Design review of the part built by this model. Coordinates are the model's own, in mm. Face numbers are marked on the shaded views. A direction names the side the tool comes from. Coordinates: 2 decimals unless noted, no trailing zeros. Write each loop counter-clockwise with the first axis right and the second up, starting at its lowest first coordinate (ties: lowest second). Pieces come first, ordered by that corner, then holes. Notation, with made-up numbers: (18.5, 67.5) - (49.5, 67.5) arc R6 ccw to (49.5, 76.5) - close; hole circle Ø4 at (-13, 50). An arc over 180 degrees is marked (long way). One line per item, written item: value.
from build123d import *

# Parameters (mm, degrees)
SKETCH5_R           = 4
SKETCH5_R_2         = 11
BOSS_EXTRUDE4_DEPTH = 10
SKETCH5_3_R         = 4
BOSS_EXTRUDE5_DEPTH = 25


with BuildPart() as part:
    # Sketch5 → Boss-Extrude4 (new body)
    with BuildSketch(Plane.XY):
        with BuildLine():
            Line((-20, 125), (-20, -125))
            ThreePointArc((-20, -125), (0, -145), (20, -125))
            Line((20, -125), (20, 125))
            ThreePointArc((20, 125), (0, 145), (-20, 125))
        make_face()
        with Locations((0, -125)):
            Circle(SKETCH5_R, mode=Mode.SUBTRACT)
        with Locations((0, 125)):
            Circle(SKETCH5_R_2, mode=Mode.SUBTRACT)
        with BuildLine():
            Line((-11, 90), (-11, -90))
            ThreePointArc((-11, -90), (0, -101), (11, -90))
            Line((11, -90), (11, 90))
            ThreePointArc((11, 90), (0, 101), (-11, 90))
        make_face(mode=Mode.SUBTRACT)
    extrude(amount=BOSS_EXTRUDE4_DEPTH)

    # Sketch5_3 → Boss-Extrude5 (add)
    with BuildSketch(Plane.XY):
        with Locations((0, -125)):
            Circle(SKETCH5_3_R)
    extrude(amount=BOSS_EXTRUDE5_DEPTH)


solid = part.part
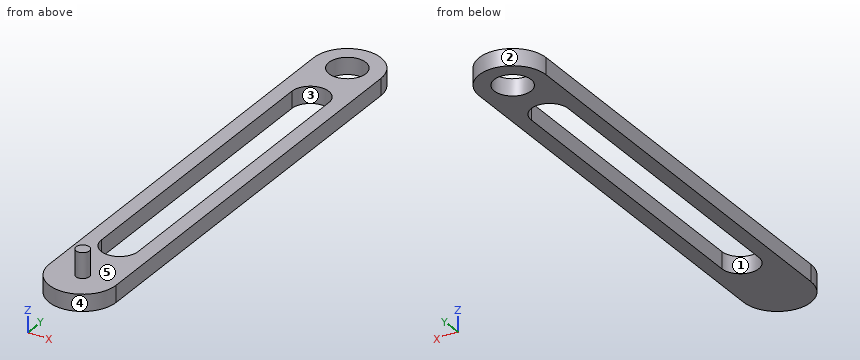
1. Consider section A-A, the plane y = -26. Write out the cut boundary in (x, z), then the cut area to 3 significant figures.
Answer block:
outline: (-20, 0) - (-11, 0) - (-11, 10) - (-20, 10) - close; (11, 0) - (20, 0) - (20, 10) - (11, 10) - close
area: 180 mm^2
2. Mouldability with a two-part tool opening along Y and no side actions: class the marked faces 3, 4 and 5 as released by +Y, released by -Y, zero draft, split by the parting line, or undercut.
Answer block:
face 3: undercut
face 4: released by -Y
face 5: zero draft
3. Consider section D-D, the plane y = 98.5. Write out the cut boundary in (x, z), then the cut area to 3 significant figures.
Answer block:
outline: (-20, 0) - (-6.98, 0) - (-6.98, 10) - (-20, 10) - close; (6.98, 0) - (20, 0) - (20, 10) - (6.98, 10) - close
area: 260 mm^2
4. Consider section C-C, the plane z = 22. Write out the cut boundary in (x, y), then the cut area to 3 significant figures.
Answer block:
outline: circle Ø8 at (0, -125)
area: 50.3 mm^2
5. Wall thickness on line 1 along Y through (x, z) = (0, 2.25); line 2 along X through (y, z) = (30.5, 3.5); line 3 along Y through (x, z) = (-5, 1.25): over which ranges is each line inside the solid? List them lowest first.
Answer block:
line 1: y = -145 to -101, 101 to 114, 136 to 145
line 2: x = -20 to -11, 11 to 20
line 3: y = -144.36 to -99.8, 99.8 to 115.2, 134.8 to 144.36
6. For the marked faces 1 and 2, list the 3-axis set-ups (+Z, -Z, +X, -X, +Y, -Y) from which the entire face can be reached by the end or side of a thin tool; tool diameter is ignored.
Answer block:
face 1: +Z, -Z
face 2: +Z, -Z, +Y
7. Consider section B-B, the plane x = 0. Write out the cut boundary in (y, z), then the cut area to 3 significant figures.
Answer block:
outline: (-145, 0) - (-101, 0) - (-101, 10) - (-121, 10) - (-121, 25) - (-129, 25) - (-129, 10) - (-145, 10) - close; (101, 0) - (114, 0) - (114, 10) - (101, 10) - close; (136, 0) - (145, 0) - (145, 10) - (136, 10) - close
area: 780 mm^2
8. Insertion check: pin 1 Ø10 at (x, z) = (-8.5, 6) entering from -Y; pin 2 Ø6 at (x, z) = (4, 5.5) entering from -Y (3 decimals); pin 3 Ø12 at (x, z) = (-10.5, 11) entering from -Y. Each pin has a flat end and moves straight along its axis. Give the tip position at first contact, or say it passes through.
Answer block:
pin 1: stops at y = -144.69
pin 2: stops at y = -144.975
pin 3: stops at y = -144.47
